```python
from build123d import *

# Parameters (mm, degrees)
F1_DEPTH = 16.764
F3_DEPTH = 6.35
F4_W     = 17.78
F4_H     = 3.81
F5_DEPTH = 3.81
F7_DEPTH = 1.27


with BuildPart() as f1:
    # F0 (on Front) → F1 (new body)
    with BuildSketch(Plane.XZ):
        Polygon((-12.7, -6.35), (0, -6.35), (12.7, -6.35), (12.7, 0), (-12.7, 0), align=None)
    extrude(amount=F1_DEPTH)

    # F2 (on face) → F3 (join)
    with BuildSketch(Plane.XY):
        Polygon((-12.7, 0), (-12.7, -16.764), (-8.89, -16.764), (-8.89, -3.81), (0, -3.81), (8.89, -3.81), (8.89, -16.764), (12.7, -16.764), (12.7, 0), align=None)
    extrude(amount=F3_DEPTH)

    # F4 (on face) → F5 (join)
    with BuildSketch(Plane.XY.offset(6.35)):
        with Locations((0, -1.905)):
            Rectangle(F4_W, F4_H)
    extrude(amount=F5_DEPTH)

    # F6 (on face) → F7 (join)
    with BuildSketch(Plane.XY.offset(6.35)):
        Polygon((-12.7, -12.954), (-12.7, -16.764), (-12.7, -20.574), (0, -20.574), (0, -12.954), align=None)
    extrude(amount=F7_DEPTH)


solid = f1.part
```
Part model, mm, in its own coordinate system. A direction names the side the tool comes from. Round coordinates to 2 decimals unless told otherwise and drop trailing zeros. Write each loop counter-clockwise with the first axis right and the second up, starting at its lowest first coordinate (ties: lowest second). Pieces come first, ordered by that corner, then holes. Notation, with made-up numbers: (63.5, 72) -> (84.5, 72) arc R16 ccw to (84.5, 85) -> close; hole circle Ø7 at (-5.75, -19.75). An arc over 180 degrees is marked (long way). Return JSON: item names as keys, results as strings. Group by question number.
Q1. Saw through at C-C on z = 5. Write the cut outline in (x, y).
Q2. Saw through at D-D on x = 6.75. Write the cut outline in (y, z).
Q3. Probe L1, parallel to X at y = -4.5, z = 3.75; L2, parallel to Z at x = 0, y = -6.5; L3, parallel to Y at x = -10.5, z = -4.75. List the from-to ranges inside material, lowest first. Write a range as [from, to].
Q4. Mould opens along Z. For faces 4 (the flat face through (-5, -17, 6.35)), 5 (the flat face through (0, -3.81, 5)), 6 (the flat face through (-6, -17, 7.62)) say: pulls with the +Z half, pulls with the -Z half, needs draft (parallel to the pull), parting line crosses it, or undercut.
Q5. Which spindle directions (+Z, -Z, +X, -X, +Y, -Y) get a long thin tool onto all of the face, cutting with end or side? Do faces 1 (the flat face through (8.89, -10, 3)), 2 (the flat face through (-6, -12.954, 7)), 3 (the flat face through (11, -8, 6.35)). Say none if no direction does.
Q6. Saw through at B-B on y = -9. Write the cut outline in (x, z), plus the area to 3 significant figures.
Q7. Pin check, flat tips, straight feed: pin 1 (8 mm diameter, centred on x = -1.5, z = 6, fed in from -Y); pin 2 (2.5 mm diameter, centred on x = -6, y = -17.5, fed in from +Z); pin 3 (4 mm diameter, centred on x = 4.5, y = -8.5, fed in from +Z); pin 4 (1.9 mm diameter, centred on x = 10.5, y = -5, fed in from +Z). Stop position of each tip, or through.
Q8. Saw through at A-A on x = -3.25. Write the cut outline in (y, z), plus the area to 3 significant figures.
Answer:
{
 "1": {"outline": "(-12.7, -16.76) -> (-8.89, -16.76) -> (-8.89, -3.81) -> (8.89, -3.81) -> (8.89, -16.76) -> (12.7, -16.76) -> (12.7, 0) -> (-12.7, 0) -> close"},
 "2": {"outline": "(-16.76, -6.35) -> (0, -6.35) -> (0, 10.16) -> (-3.81, 10.16) -> (-3.81, 0) -> (-16.76, 0) -> close"},
 "3": {"L1": "[-12.7, -8.89], [8.89, 12.7]", "L2": "[-6.35, 0]", "L3": "[-16.76, 0]"},
 "4": {"face 4": "undercut", "face 5": "needs draft", "face 6": "pulls with the +Z half"},
 "5": {"face 1": "+Z, -Y", "face 2": "+Z, +X, -X", "face 3": "+Z, +X, +Y, -Y"},
 "6": {"outline": "(-12.7, -6.35) -> (12.7, -6.35) -> (12.7, 6.35) -> (8.89, 6.35) -> (8.89, 0) -> (-8.89, 0) -> (-8.89, 6.35) -> (-12.7, 6.35) -> close", "area": "210 mm2"},
 "7": {"pin 1": "y = -20.57", "pin 2": "z = 7.62", "pin 3": "z = 0", "pin 4": "z = 6.35"},
 "8": {"outline": "(-20.57, 6.35) -> (-12.95, 6.35) -> (-12.95, 7.62) -> (-20.57, 7.62) -> close; (-16.76, -6.35) -> (0, -6.35) -> (0, 10.16) -> (-3.81, 10.16) -> (-3.81, 0) -> (-16.76, 0) -> close", "area": "155 mm2"}
}
